from build123d import *

# Parameters (mm, degrees)
F1_DEPTH = 5.6642
F3_DEPTH = 1.524
F4_DEPTH = 1.524
F6_DEPTH = 9.2964
F7_R     = 0.762
F8_R     = 1.9431
F9_DEPTH = 12.7


with BuildPart() as f1:
    # F0 (on Top) → F1 (new body)
    with BuildSketch(Plane.XY):
        with BuildLine():
            Line((4.1529, -5.6261), (4.1529, 0))
            ThreePointArc((4.1529, 0), (0, 4.1529), (-4.1529, 0))
            Line((-4.1529, 0), (-4.1529, -5.6261))
            Line((-4.1529, -5.6261), (4.1529, -5.6261))
        make_face()
    extrude(amount=-F1_DEPTH)

    # F2 (on face) → F3 (join)
    with BuildSketch(Plane.XY):
        with BuildLine():
            ThreePointArc((5.0419, 0), (0, 5.0419), (-5.0419, 0))
            Line((-5.0419, 0), (-5.0419, -6.5151))
            Line((-5.0419, -6.5151), (5.0419, -6.5151))
            Line((5.0419, -6.5151), (5.0419, 0))
        make_face()
        with BuildLine():
            Line((-4.1529, -5.6261), (-4.1529, 0))
            ThreePointArc((-4.1529, 0), (0, 4.1529), (4.1529, 0))
            Line((4.1529, 0), (4.1529, -5.6261))
            Line((4.1529, -5.6261), (-4.1529, -5.6261))
        make_face(mode=Mode.SUBTRACT)
    extrude(amount=F3_DEPTH)



with BuildPart() as f4:
    # F1_face (on face) → F4 (new body, through all)
    with BuildSketch(Plane(origin=(0, -1.133876, 0), x_dir=(1, 0, 0), z_dir=(0, 0, 1))):
        with BuildLine():
            Line((-4.1529, 1.133876), (-4.1529, -4.492224))
            Line((-4.1529, -4.492224), (4.1529, -4.492224))
            Line((4.1529, -4.492224), (4.1529, 1.133876))
            ThreePointArc((4.1529, 1.133876), (0, 5.286776), (-4.1529, 1.133876))
        make_face()
    extrude(amount=F4_DEPTH)


with BuildPart() as f1_1:
    add(f1.part)

    add(f4.part)  # F6 merges F4
    # F5 (on face) → F6 (join)
    with BuildSketch(Plane.XZ.offset(5.6261)):
        with BuildLine():
            ThreePointArc((-2.444742, 0), (-0.970892, -4.744129), (3.0607, -1.8415))
            ThreePointArc((3.0607, -1.8415), (2.902629, -0.870608), (2.444742, 0))
            Line((2.444742, 0), (-2.444742, 0))
        make_face()
        with BuildLine():
            Line((-2.444742, 0), (2.444742, 0))
            ThreePointArc((2.444742, 0), (0, 1.2192), (-2.444742, 0))
        make_face()
    extrude(amount=F6_DEPTH)

    # F7
    f7_edges = [f1_1.edges().sort_by_distance(p)[0] for p in [
        (5.0419, -3.25755, 1.524),
    ]]
    fillet(f7_edges, radius=F7_R)

    # F8 (on face) → F9 (join)
    with BuildSketch(Plane.XZ.offset(14.9225)):
        with Locations((0, -1.8415)):
            Circle(F8_R)
    extrude(amount=F9_DEPTH)


solid = f1_1.part
Verification items for the finished model (mm, model axes). A direction names the side the tool comes from. Coordinates: 2 decimals unless noted, no trailing zeros. Order: outer loops, then holes, each group sorted by start corner. A loop starts at its lowest first (then second) coordinate and runs counter-clockwise, first axis right, second up.
Item 1: Material ranges on L1, parallel to X at y = -5, z = -1; L2, parallel to Y at x = 0, z = -0.5; L3, parallel to X at y = -17, z = -0.5, recorded low to high.
Filled in:
L1: x = -4.15 to 4.15
L2: y = -27.62 to 4.15
L3: x = -1.41 to 1.41
Item 2: Section check A-A, the plane x = 0. Enter the section's corners in (y, z).
Filled in:
outline: (-27.62, -3.78) - (-14.92, -3.78) - (-14.92, -4.9) - (-5.63, -4.9) - (-5.63, -5.66) - (4.15, -5.66) - (4.15, 0) - (5.04, 0) - (5.04, 0.76) arc R0.76 ccw to (4.28, 1.52) - (-6.52, 1.52) - (-6.52, 1.22) - (-14.92, 1.22) - (-14.92, 0.1) - (-27.62, 0.1) - close
Item 3: Section check C-C, the plane z = -1.5. Enter the section's corners in (x, y), then the cut area to 3 significant figures.
Filled in:
outline: (-4.15, -5.63) - (-3.04, -5.63) - (-3.04, -14.92) - (-1.91, -14.92) - (-1.91, -27.62) - (1.91, -27.62) - (1.91, -14.92) - (3.04, -14.92) - (3.04, -5.63) - (4.15, -5.63) - (4.15, 0) arc R4.15 ccw to (-4.15, 0) - close
area: 179 mm2
Item 4: Section check B-B, the plane y = -4. Enter the section's corners in (x, z).
Filled in:
outline: (-5.04, 0) - (-4.15, 0) - (-4.15, -5.66) - (4.15, -5.66) - (4.15, 0) - (5.04, 0) - (5.04, 0.76) arc R0.76 ccw to (4.28, 1.52) - (-4.28, 1.52) arc R0.76 ccw to (-5.04, 0.76) - close
Item 5: Access from +Z, -Z, +X, -X, +Y, -Y to the whole of each face (thin tool, end or side, straight path). Record for faces 1 (the face through (-1.2, -6.515, 1.3)), 2 (the face through (0.09, 4.15, -2.79)), 3 (the face through (-4.153, -3, -3)), 4 (the face through (0, -14.922, -4)), 5 (the face through (4.153, -3, -3)).
Filled in:
face 1: +Z, -Y
face 2: -Z, +Y
face 3: -Z, -X, +Y, -Y
face 4: -Y
face 5: -Z, +X, +Y, -Y
Item 6: Depth check by flat-ended pin: pin 1 (1.7 mm diameter, centred on x = -2, z = 1, fed in from -Y); pin 2 (5 mm diameter, centred on x = -0.5, y = -12, fed in from -Z); pin 3 (1.5 mm diameter, centred on x = 2.5, y = -7, fed in from -Z). Enter the tip coordinate at first touch or a pass-through.
Filled in:
pin 1: stops at y = -14.92
pin 2: stops at z = -4.9
pin 3: stops at z = -4.35
Item 7: Section check D-D, the plane y = -20. Enter the section's corners in (x, z), then the cut area to 3 significant figures.
Filled in:
outline: circle Ø3.89 at (0, -1.84)
area: 11.9 mm2
